Geometry: see drawing. Coordinates: mm, zero at the bounding-box minimum. A direction names the side the tool comes from. Give positions to 0.01 mm unless a question says otherwise; leave off trailing zeros. Order: outer loops, then holes, each group sorted by start corner. A loop starts at its lowest first (then second) coordinate and runs counter-clockwise, first axis right, second up. Notation, with made-up numbers: M 29.25,-33.75 L 62.25,-33.75 A12 ccw 62.25,-10.75 Z; hole C 29,70.25 d10. An arc over 180 degrees is marked long. Return JSON: item names as keys, results as strings.
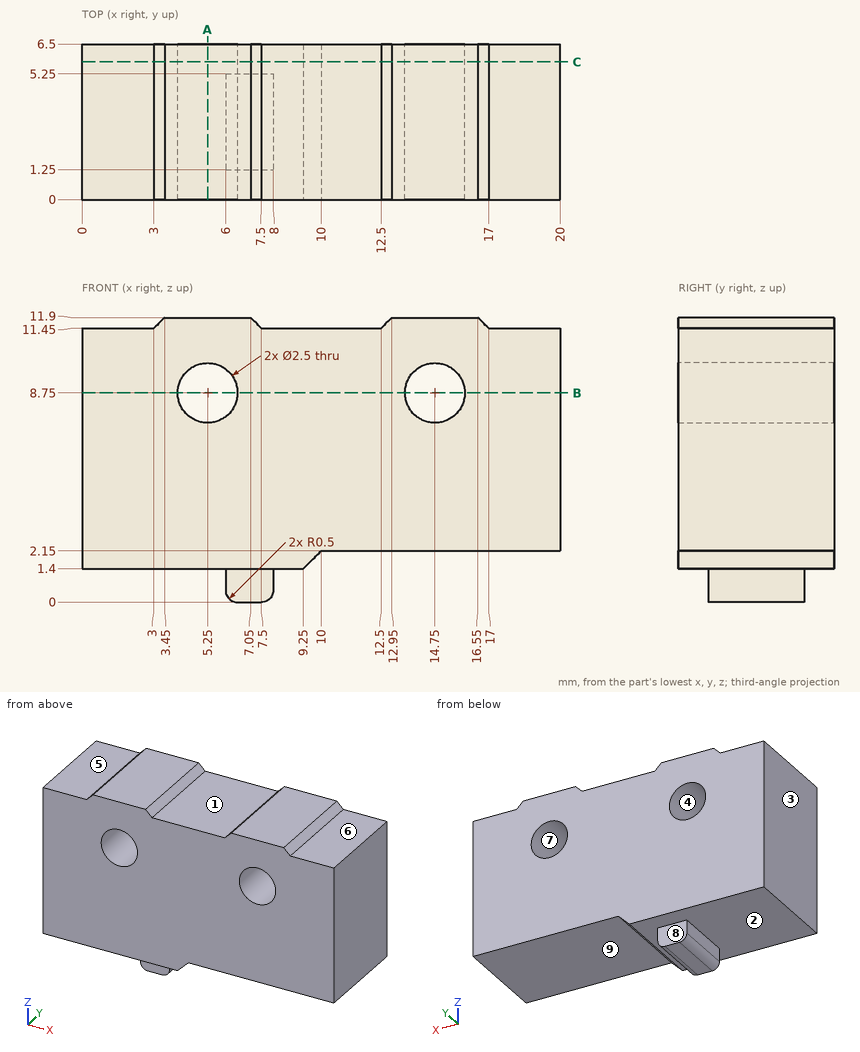
1. Section query A-A (x = 5.25). Return loops of the section in (y, z).
Evaluation:
{"outline": "M 0,1.4 L 6.5,1.4 L 6.5,7.5 L 0,7.5 Z; M 0,10 L 6.5,10 L 6.5,11.9 L 0,11.9 Z"}
2. First-contact query: pin 1 (0.7 mm diameter, centred on x = 7, z = 0.5, fed in from +Y); pin 2 (1.1 mm diameter, centred on x = 7.5, z = 0.5, fed in from -Y); pin 3 (0.7 mm diameter, centred on y = 3, z = 1, fed in from -X); pin 4 (2 mm diameter, centred on x = 14.75, z = 8.75, fed in from -Y). Flat tips, straight axial feed; report the tip coordinate or a pass-through.
Evaluation:
{"pin 1": "stops at y = 5.25", "pin 2": "stops at y = 1.25", "pin 3": "stops at x = 6", "pin 4": "passes through"}
3. Draft query along X for the marked faces 1, 2, 3 and 4. Return one class per face: pulls with the +X half, pulls with the -X half, needs draft (parallel to the pull), parting line crosses it, or undercut.
Evaluation:
{"face 1": "undercut", "face 2": "needs draft", "face 3": "pulls with the -X half", "face 4": "undercut"}
4. Ray query, probe 1 along X at (y, z) = (4.25, 8.75); probe 2 along X at (y, z) = (6.25, 8.25); probe 3 along X at (y, z) = (2.5, 1). Return the intervals inside material, ascending.
Evaluation:
{"probe 1": "x = 0 to 4, 6.5 to 13.5, 16 to 20", "probe 2": "x = 0 to 4.1, 6.4 to 13.6, 15.9 to 20", "probe 3": "x = 6 to 8"}
5. Section query C-C (y = 5.75). State how many separate pieces and enclosed holes the cut face has, then the cut area to 3 significant figures.
Evaluation:
{"separate pieces": "1", "enclosed holes": "2", "area": "187 mm^2"}
6. Set-up query: the marked faces 5, 6, 7, 8 and 9. Return all of +Z, -Z, +X, -X, +Y, -Y with unobstructed straight access to the full face (end or side cutting, diameter ignored); none if empty.
Evaluation:
{"face 5": "+Z, -X, +Y, -Y", "face 6": "+Z, +X, +Y, -Y", "face 7": "+Y, -Y", "face 8": "-Z, +X, -X, +Y", "face 9": "-Z, +X, +Y, -Y"}
7. Section query B-B (z = 8.75). Return loops of the section in (x, y).
Evaluation:
{"outline": "M 0,0 L 4,0 L 4,6.5 L 0,6.5 Z; M 6.5,0 L 13.5,0 L 13.5,6.5 L 6.5,6.5 Z; M 16,0 L 20,0 L 20,6.5 L 16,6.5 Z"}
